For this review, take the finished solid that the model builds, in its own axes (mm). A direction names the side the tool comes from. Round coordinates to 2 decimals unless told otherwise and drop trailing zeros. Write each loop counter-clockwise with the first axis right and the second up, starting at its lowest first coordinate (ties: lowest second). Pieces come first, ordered by that corner, then holes. Notation, with made-up numbers: (30.5, -35.5) -> (60.5, -35.5) arc R20 cw to (60.5, -15.5) -> close; hole circle Ø3 at (54, 14.5). An arc over 180 degrees is marked (long way). Answer in a Markdown table with one row per item.
from build123d import *

# Parameters (mm, degrees)
F0_W     = 101.6
F0_H     = 76.2
F1_DEPTH = 50.8
F3_DEPTH = 25.4
F5_DEPTH = 25.4


with BuildPart() as f1:
    # F0 (on Top) → F1 (new body)
    with BuildSketch(Plane.XY):
        with Locations((10.068508, -14.225589)):
            Rectangle(F0_W, F0_H)
    extrude(amount=F1_DEPTH)

    # F2 (on face) → F3 (cut)
    with BuildSketch(Plane.XY.offset(50.8)):
        Polygon((-40.731492, -52.325589), (35.468508, -52.325589), (60.868508, -14.225589), (60.868508, 23.874411), (-40.731492, 23.874411), align=None)
    extrude(amount=-F3_DEPTH, mode=Mode.SUBTRACT)

    # F4 (on face) → F5 (join)
    with BuildSketch(Plane.XY.offset(25.4)):
        Polygon((-40.731492, 23.874411), (-40.731492, -52.325589), (-28.031492, -52.325589), (22.768508, 23.874411), align=None)
    extrude(amount=F5_DEPTH)


solid = f1.part
1) Clearance check with a flat-ended pin moving along its axis: pin 1 Ø3 at (x, z) = (19.5, 43) entering from -Y. State where the tip first meets the part, or that it passes through.
Solved:
| item | result |
|---|---|
| pin 1 | y = 16.72 |
2) For line 1 (Z direction, x = 29.5, y = -4); line 2 (X direction, y = -36, z = 29); line 3 (X direction, y = -12, z = 36), list the stretches that pass through material, from the lowest coordinate up. Write a range as [from, to].
Solved:
| item | result |
|---|---|
| line 1 | [0, 25.4] |
| line 2 | [-40.73, -17.15], [46.35, 60.87] |
| line 3 | [-40.73, -1.15] |
3) For faces 1 (the flat face through (-16, -5, 50.8)), 2 (the flat face through (47.99, -33.54, 38.28)), 3 (the flat face through (-2.99, -14.76, 37.92)), list the 3-axis set-ups (+Z, -Z, +X, -X, +Y, -Y) from which the entire face can be reached by the end or side of a thin tool; tool diameter is ignored.
Solved:
| item | result |
|---|---|
| face 1 | +Z, +X, -X, +Y, -Y |
| face 2 | +Z, +Y |
| face 3 | +Z, -Y |
4) Consider section D-D on x = 26.5. State the section outline as (y, z) points.
Solved:
| item | result |
|---|---|
| outline | (-52.33, 0) -> (23.87, 0) -> (23.87, 25.4) -> (-52.33, 25.4) -> close |
5) Consider section C-C on x = 2. State the section outline as (y, z) points.
Solved:
| item | result |
|---|---|
| outline | (-52.33, 0) -> (23.87, 0) -> (23.87, 50.8) -> (-7.28, 50.8) -> (-7.28, 25.4) -> (-52.33, 25.4) -> close |
6) Mouldability with a two-part tool opening along X and no side actions: class faces 4 (the flat face through (-40.731, -14, 25)), 5 (the flat face through (26, -14, 25.4)), 6 (the flat face through (9, -14, 0)) as pulls with the +X half, pulls with the -X half, needs draft (parallel to the pull), parting line crosses it, or undercut.
Solved:
| item | result |
|---|---|
| face 4 | pulls with the -X half |
| face 5 | undercut |
| face 6 | needs draft |
7) Consider section B-B on y = -10.5. State the section outline as (x, z) points.
Solved:
| item | result |
|---|---|
| outline | (-40.73, 0) -> (60.87, 0) -> (60.87, 25.4) -> (-0.15, 25.4) -> (-0.15, 50.8) -> (-40.73, 50.8) -> close |
8) Consider section A-A on z = 30.5. State the section outline as (x, y) points.
Solved:
| item | result |
|---|---|
| outline | (-40.73, -52.33) -> (-28.03, -52.33) -> (22.77, 23.87) -> (-40.73, 23.87) -> close; (35.47, -52.33) -> (60.87, -52.33) -> (60.87, -14.23) -> close |
